Input: dimensioned drawing with shaded views. Units: mm. Origin: part minimum x, y, z. A direction names the side the tool comes from. Coordinates: 2 decimals unless noted, no trailing zeros. Order: outer loops, then holes, each group sorted by start corner. A loop starts at its lowest first (then second) coordinate and runs counter-clockwise, first axis right, second up. Notation, with made-up numbers: M -31,-18.75 L 1,-18.75 A10 cw 1,-13.75 Z; hole C -2.75,-33 d6. An arc over 180 degrees is marked long. Write item = value, one per line.
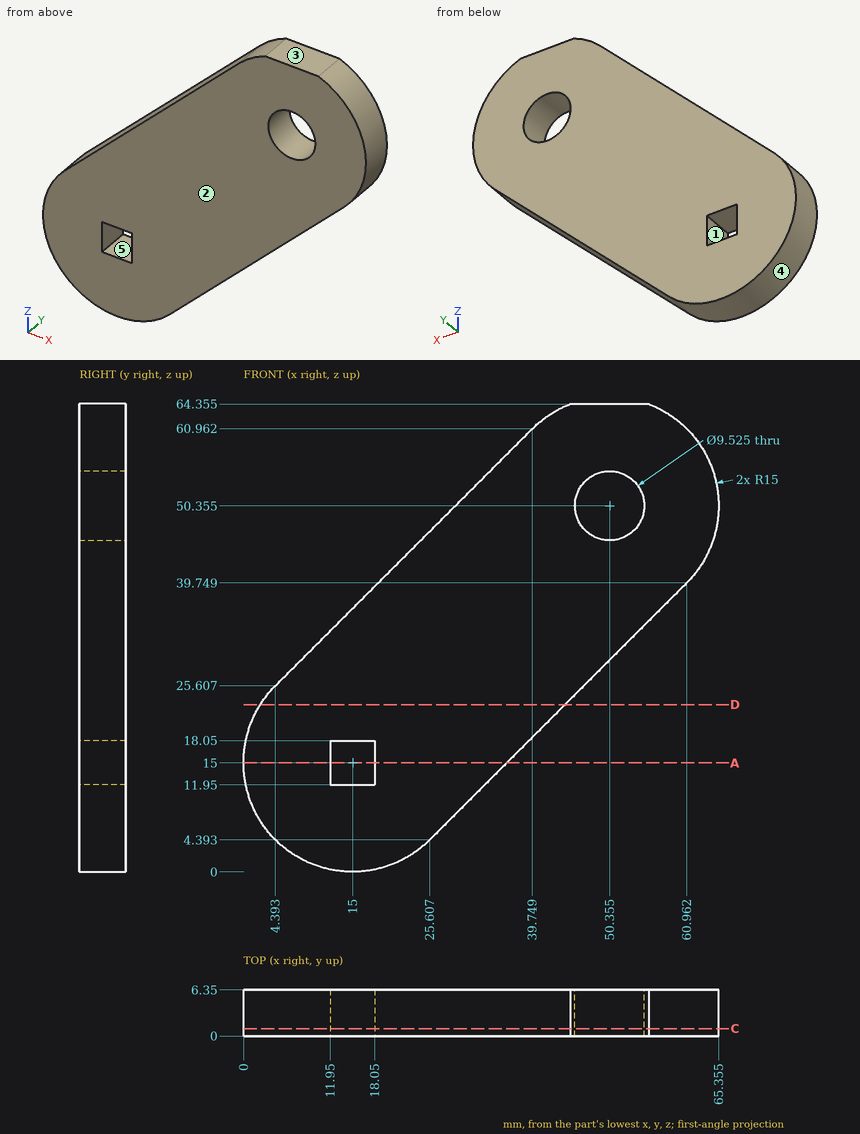
1) Line query: L1, parallel to X at y = 4, z = 50.5 (1 decimal); L2, parallel to X at y = 5.25, z = 51 (1 decimal); L3, parallel to Z at x = 42, y = 0.75 (1 decimal). Output: solid intervals per line, ascending.
Numbers:
L1 = 29.3 to 45.6, 55.1 to 65.4
L2 = 29.8 to 45.6, 55.1 to 65.3
L3 = 20.8 to 62.8
2) Set-up query: the marked faces 1 and 2. Return all of +Z, -Z, +X, -X, +Y, -Y with unobstructed straight access to the full face (end or side cutting, diameter ignored); none if empty.
Numbers:
face_1 = +Y, -Y
face_2 = +Z, -Z, +X, -X, -Y
3) Section C-C, the plane y = 1. Give the number of separate pieces and of enclosed holes in the cut face, and give its area (3 significant figures).
Numbers:
separate_pieces = 1
enclosed_holes = 2
area = 2,090 mm²
4) Section A-A, the plane z = 15. Return loops of the section in (x, y), and give its area (3 significant figures).
Numbers:
outline = M 0,0 L 11.95,0 L 11.95,6.35 L 0,6.35 Z; M 18.05,0 L 36.21,0 L 36.21,6.35 L 18.05,6.35 Z
area = 191 mm²
5) Mould query, pull axis X, two halves, no side actions, for the marked faces 3, 4 and 5. Classes: pulls with the +X half, pulls with the -X half, needs draft (parallel to the pull), parting line crosses it, or undercut.
Numbers:
face_3 = needs draft
face_4 = parting line crosses it
face_5 = undercut
6) Pin query (flat end, axial travel): pin 1 (1.5 mm diameter, centred on y = 1, z = 28, fed in from -X); pin 2 (2 mm diameter, centred on y = 1, z = 19.5, fed in from -X); pin 3 (1.5 mm diameter, centred on x = 31.5, y = 1, fed in from -Z). Return the tip coordinate at first contact, or that it passes through.
Numbers:
pin_1 = 6.04
pin_2 = 0.41
pin_3 = 9.54
7) Section D-D, the plane z = 23. Return loops of the section in (x, y), and give its area (3 significant figures).
Numbers:
outline = M 2.31,0 L 44.21,0 L 44.21,6.35 L 2.31,6.35 Z
area = 266 mm²
